Source: CAD feature listing. Evaluate the final solid. Frame: model axes, mm. A direction names the side the tool comes from. Give positions to 0.01 mm unless a question says otherwise; leave off trailing zeros. Loops run counter-clockwise (first coordinate to the right, second up) from the corner with the lowest first, then second, coordinate; pieces in that order, holes last. Notation, with made-up numbers: (-14.75, 16.5) - (23.25, 16.5) arc R23 cw to (23.25, 33.5) - close; hole circle Ø7 at (-27.75, 80). An arc over 180 degrees is marked (long way). Write each question's results on one line, items separated by ' | '. Start each with the question number.
(1) Pull-direction query (Y, two-part tool) for faces 3 (the flat face through (2, -1, 3)), 4 (the cylindrical face through (2.685, 0.596, 0.384)), 5 (the cylindrical face through (2, 0, 0)); classes: pulls with the +Y half, pulls with the -Y half, needs draft (parallel to the pull), parting line crosses it, or undercut.
(2) Reachability of faces 1 (the flat face through (1, 2, -3)), 2 (the flat face through (3, 0, -2.25)) from +Z, -Z, +X, -X, +Y, -Y: full face, straight path, thin tool, end or side. Return the list, or none.
(3) Contact query for flat-ended pins moving along their axis: pin 1 (1 mm diameter, centred on y = -1, z = -0.5, fed in from -X); pin 2 (3 mm diameter, centred on x = -1.5, y = -3, fed in from +Z); pin 3 (3.5 mm diameter, centred on x = 0, y = 0, fed in from +Z) (3 decimals). Output: stop coordinate, or through.
(4) Cut plane A-A on y = 0. Return the cut outline in (x, z), then the cut area to 3 significant figures.
(5) Cut plane C-C on z = -1.25. Return the cut outline in (x, y).
(6) Material intervals for line 1 along Y through (x, z) = (0, -1.6); line 2 along Z through (x, y) = (-3.25, -2), sorted ascending. Write a range as [from, to].
from build123d import *

# Parameters (mm, degrees)
CHAMFER1_SIZE = 0.1125
CHAMFER2_SIZE = 0.0375
FILLET1_R     = 0.06


with BuildPart() as part:
    # Sketch3 → Revolve1 (revolve)
    with BuildSketch(Plane(origin=(0, 0, 0), x_dir=(0, 0, -1), z_dir=(1, 0, 0))):
        Polygon((3, -4.75), (2.25, -4.75), (2.25, -2.75), (-3, -2.75), (-3, -2), (3, -2), align=None)
    revolve(axis=Axis((0, 0, 3), (0, 0, -1)))

    # Chamfer1
    chamfer1_edges = [part.edges().sort_by_distance(p)[0] for p in [
        (0, 2.75, 3),
    ]]
    chamfer(chamfer1_edges, length=CHAMFER1_SIZE)

    # Chamfer2
    chamfer2_edges = [part.edges().sort_by_distance(p)[0] for p in [
        (0, 2, -3),
        (0, 2, 3),
    ]]
    chamfer(chamfer2_edges, length=CHAMFER2_SIZE)

    # Fillet1
    fillet1_edges = [part.edges().sort_by_distance(p)[0] for p in [
        (0, 2.75, -2.25),
        (0, 4.75, -2.25),
        (0, 4.75, -3),
    ]]
    fillet(fillet1_edges, radius=FILLET1_R)


solid = part.part
Ans:
1) face 3: needs draft | face 4: parting line crosses it | face 5: undercut
2) face 1: -Z, +X, -X, +Y, -Y | face 2: +Z
3) pin 1: x = -2.7 | pin 2: z = 3 | pin 3: through
4) outline: (-4.75, -2.94) arc R0.06 ccw to (-4.69, -3) - (-2.04, -3) - (-2, -2.96) - (-2, 2.96) - (-2.04, 3) - (-2.64, 3) - (-2.75, 2.89) - (-2.75, -2.19) arc R0.06 cw to (-2.81, -2.25) - (-4.69, -2.25) arc R0.06 ccw to (-4.75, -2.31) - close; (2, -2.96) - (2.04, -3) - (4.69, -3) arc R0.06 ccw to (4.75, -2.94) - (4.75, -2.31) arc R0.06 ccw to (4.69, -2.25) - (2.81, -2.25) arc R0.06 cw to (2.75, -2.19) - (2.75, 2.89) - (2.64, 3) - (2.04, 3) - (2, 2.96) - close | area: 12.0 mm^2
5) outline: circle Ø5.5 at (0, 0); hole circle Ø4 at (0, 0)
6) line 1: [-2.75, -2], [2, 2.75] | line 2: [-3, -2.25]
